Input: dimensioned drawing with shaded views. Units: mm. Origin: part minimum x, y, z. Round coordinates to 2 decimals unless told otherwise and drop trailing zeros. Write each loop counter-clockwise with the first axis right and the second up, starting at its lowest first coordinate (ties: lowest second). Pieces come first, ordered by that corner, then holes. Notation, with made-up numbers: M 26,21.25 L 83,21.25 A11 ccw 83,29.25 Z; hole C 11.5,41 d8. An arc over 180 degrees is marked long. Put each result on its own line as item: value. Start each with the question number.
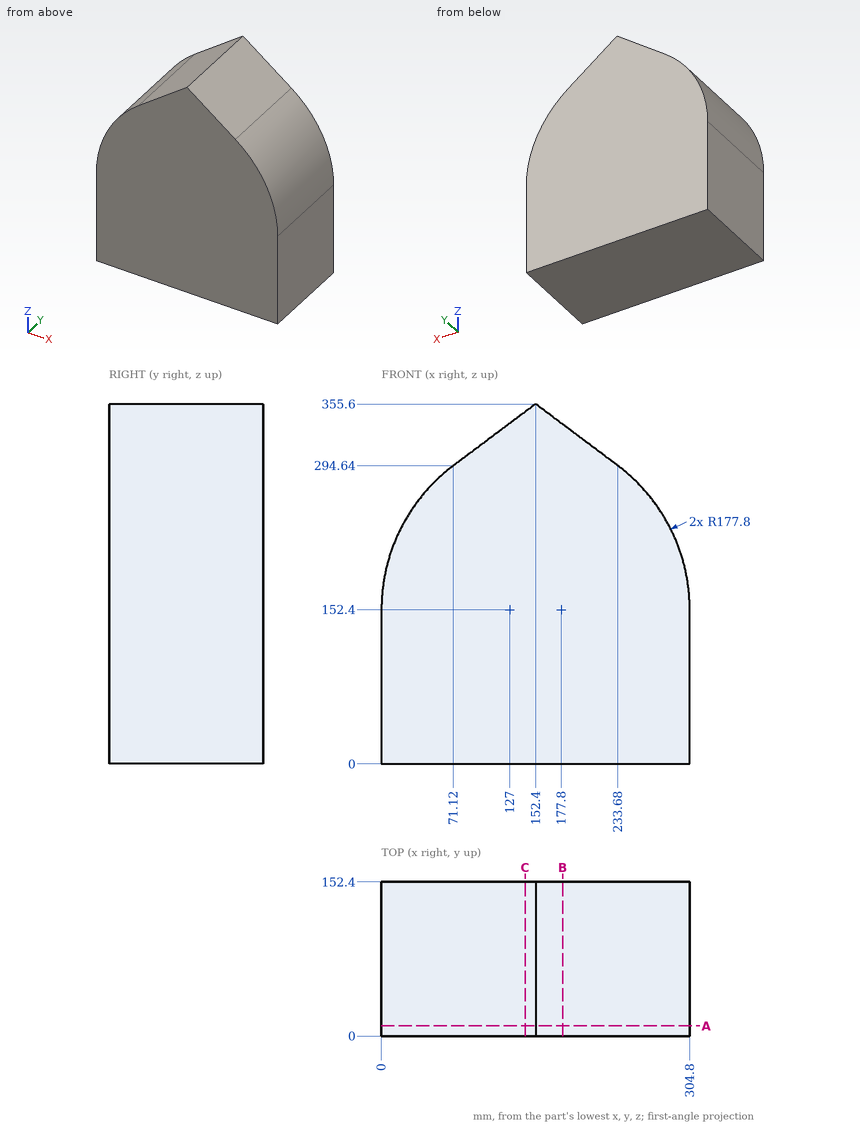
1) Section C-C, the plane x = 142. Output: boundary loops of the cut face in (y, z).
2) First-contact query: pin 1 (4 mm diameter, centred on x = 59, y = 24, fed in from +Z); pin 2 (2 mm diameter, centred on y = 26, z = 157.5, fed in from +X); pin 3 (4 mm diameter, centred on x = 63.5, y = 97, fed in from -Z); pin 4 (8 mm diameter, centred on y = 18.5, z = 205.5, fed in from -X). Flat tips, straight axial feed; report the tip coordinate or a pass-through.
3) Section B-B, the plane x = 179. Output: boundary loops of the cut face in (y, z).
4) Ray query, probe 1 along X at (y, z) = (108.5, 156.5); probe 2 along X at (y, z) = (41, 305); probe 3 along Z at (x, y) = (19.5, 23.5). Return the intervals inside material, ascending.
5) Section A-A, the plane y = 10. Output: boundary loops of the cut face in (x, z).
Solved:
1. outline: M 0,0 L 152.4,0 L 152.4,347.8 L 0,347.8 Z
2. pin 1: stops at z = 286.45
2. pin 2: stops at x = 304.75
2. pin 3: stops at z = 0
2. pin 4: stops at x = 6.91
3. outline: M 0,0 L 152.4,0 L 152.4,335.65 L 0,335.65 Z
4. probe 1: x = 0.05 to 304.75
4. probe 2: x = 84.93 to 219.87
4. probe 3: z = 0 to 233.36
5. outline: M 0,0 L 304.8,0 L 304.8,152.4 A177.8 ccw 233.68,294.64 L 152.4,355.6 L 71.12,294.64 A177.8 ccw 0,152.4 Z
